from build123d import *

# Parameters (mm, degrees)
SKETCH1_W           = 50
SKETCH1_H           = 50
SKETCH1_R           = 20.5
BOSS_EXTRUDE1_DEPTH = 20
SKETCH2_W           = 20
SKETCH2_H           = 50
BOSS_EXTRUDE2_DEPTH = 20
CUT_EXTRUDE1_DEPTH  = 20
BOSS_EXTRUDE3_DEPTH = 20
FILLET1_R           = 10


with BuildPart() as part:
    # Sketch1 → Boss-Extrude1 (new body)
    with BuildSketch(Plane.XY):
        Rectangle(SKETCH1_W, SKETCH1_H)
        Circle(SKETCH1_R, mode=Mode.SUBTRACT)
    extrude(amount=BOSS_EXTRUDE1_DEPTH)

    # Sketch2 → Boss-Extrude2 (add)
    with BuildSketch(Plane.ZY.offset(25)):
        with Locations((10, 0)):
            Rectangle(SKETCH2_W, SKETCH2_H)
    extrude(amount=BOSS_EXTRUDE2_DEPTH)

    # Sketch3 → Cut-Extrude1 (cut)
    with BuildSketch(Plane.XY.offset(20)):
        with BuildLine():
            Line((-45, 25), (-45, 10))
            add(Edge.make_bspline(
                [(-45, 10), (-25.372837907, 9.072160547), (-10, 25)],
                knots=[0, 0, 0, 1, 1, 1], degree=2))
            Line((-10, 25), (-45, 25))
        make_face()
        with BuildLine():
            add(Edge.make_bspline(
                [(-45, -10), (-25.372837907, -9.072160547), (-10, -25)],
                knots=[0, 0, 0, 1, 1, 1], degree=2))
            Line((-45, -10), (-45, -25))
            Line((-45, -25), (-10, -25))
        make_face()
    extrude(amount=-CUT_EXTRUDE1_DEPTH, mode=Mode.SUBTRACT)

    # Sketch4 → Boss-Extrude3 (add)
    with BuildSketch(Plane.XY.offset(20)):
        Polygon((-46.455, -3.125), (-45, -3.125), (-45, 3.125), (-46.455, 3.125), (-46.8, 3.125), (-47.3, 3.125), (-47.3, 5.5), (-48.439339828, 5.5), (-51.1, 2.839339828), (-51.1, 0.21), (-51.31, 0), (-51.1, -0.21), (-51.1, -2.839339828), (-48.439339828, -5.5), (-47.3, -5.5), (-47.3, -3.125), (-46.8, -3.125), align=None)
    extrude(amount=-BOSS_EXTRUDE3_DEPTH)

    # Fillet1
    fillet1_edges = [part.edges().sort_by_distance(p)[0] for p in [
        (25, -25, 10),
        (25, 25, 10),
    ]]
    fillet(fillet1_edges, radius=FILLET1_R)


solid = part.part
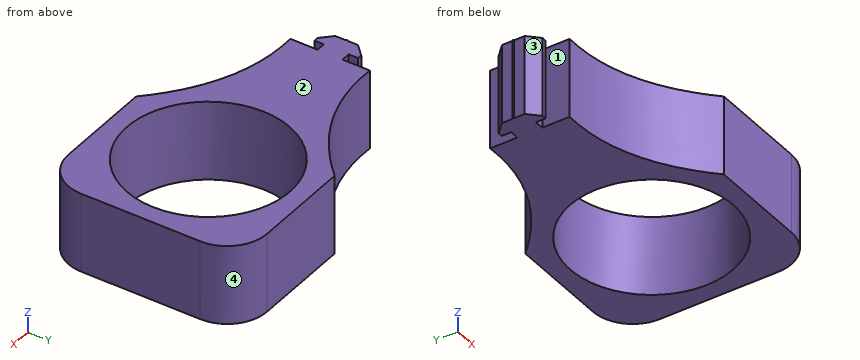
Could you check a few things on this model? Use its own coordinates, in mm. Face numbers are marked on the shaded views. Round coordinates to 2 decimals unless told otherwise and drop trailing zeros. Write each loop counter-clockwise with the first axis right and the second up, starting at its lowest first coordinate (ties: lowest second). Pieces come first, ordered by that corner, then holes. Notation, with made-up numbers: (20, 6) - (30, 6) arc R11 ccw to (30, 25) - close; hole circle Ø11 at (63, 20.25). An arc over 180 degrees is marked (long way). Use a Markdown table: item, result.
Q1. For pin 1 (1.1 mm diameter, centred on x = -46.5, z = 11, fed in from -Y) (3 decimals); pin 2 (8 mm diameter, centred on x = -16, z = 16.5, fed in from +Y); pin 3 (1.3 mm diameter, centred on x = -48, z = 13, fed in from -Y), each with a flat end and sliding along its axis, tell me the tip position at first contact or that it passes through.
Output values:
| item | result |
|---|---|
| pin 1 | y = -3.125 |
| pin 2 | y = 23.02 |
| pin 3 | y = -5.5 |
Q2. I want a section at B-B (y = -8). List the corners of the cut face in (x, z) for me, plus the area to 3 significant figures.
Output values:
| item | result |
|---|---|
| outline | (-45, 0) - (-18.87, 0) - (-18.87, 20) - (-45, 20) - close; (18.87, 0) - (25, 0) - (25, 20) - (18.87, 20) - close |
| area | 645 mm2 |
Q3. I want a section at A-A (x = 0). List the corners of the cut face in (y, z) for me.
Output values:
| item | result |
|---|---|
| outline | (-25, 0) - (-20.5, 0) - (-20.5, 20) - (-25, 20) - close; (20.5, 0) - (25, 0) - (25, 20) - (20.5, 20) - close |
Q4. Thinking about a two-plate mould opening in X: for the marked faces 1, 2, 3 and 4, which applies, released by +X, released by -X, zero draft, split by the parting line, or undercut?
Output values:
| item | result |
|---|---|
| face 1 | undercut |
| face 2 | zero draft |
| face 3 | released by -X |
| face 4 | released by +X |
Q5. Please list where these lines run through material, in increasing order: L1, parallel to Y at x = 0, z = 13.5; L2, parallel to X at y = 5, z = 12.75; L3, parallel to Y at x = -44.5, z = 12.75.
Output values:
| item | result |
|---|---|
| L1 | -25 to -20.5, 20.5 to 25 |
| L2 | -48.94 to -47.3, -45 to -19.88, 19.88 to 25 |
| L3 | -9.98 to 9.98 |
